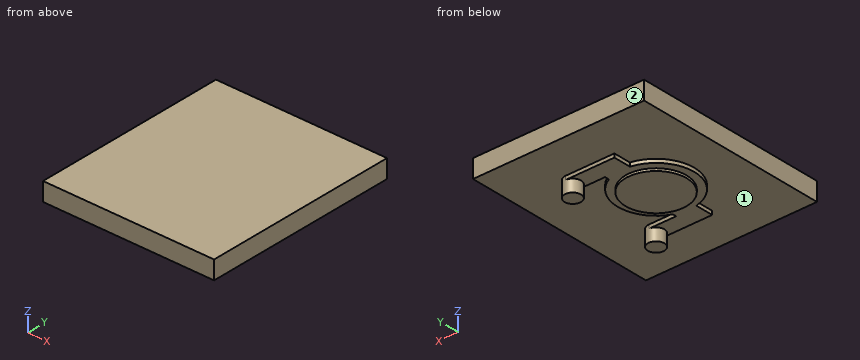
Autodesk Inventor part; units mm, degrees
ref_plane "Work Plane2" through (-8.091, -6.214, -0.6) normal (0, 0, 1) x (1, 0, 0)
ref_plane "Work Plane3" through (-9, -11.7, -1) normal (0, 0, -1) x (0, 1, 0)
ref_plane "YZ Plane" through (0, 0, 0) normal (1, 0, 0) x (0, 1, 0)
ref_plane "Work Plane1" through (0, 0, 0) normal (0, 0, 1) x (1, 0, 0)
sketch "Sketch1" plane through (0, 0, 0) normal (0, 0, 1) x (1, 0, 0)
  line L0 (9, 11.7) -> (-9, 11.7)
  line L1 (-9, 11.7) -> (-9, -11.7)
  line L2 (-9, -11.7) -> (9, -11.7)
  line L3 (9, -11.7) -> (9, 11.7)
  line L4 (5, -9.05) -> (-2.9937, -9.05)
  line L5 (-2.9937, -9.05) -> (-2.9937, -6.1068)
  arc A0 (-2.9937, 6.1788) -> (-2.9937, -6.1068) centre (-1.841, 0.036) ccw
  line L6 (-2.9937, 6.1788) -> (-2.9937, 9.05)
  line L7 (-2.9937, 9.05) -> (5, 9.05)
  arc A1 (5, 6.35) -> (5, 9.05) centre (5, 7.7) ccw
  line L8 (5, 6.35) -> (0.9246, 6.35)
  line L9 (0.9246, 6.35) -> (0.9246, 5.6409)
  arc A2 (0.5216, -5.7502) -> (0.9246, 5.6409) centre (-1.841, 0.036) ccw
  line L10 (0.5216, -5.7502) -> (0.5216, -6.35)
  line L11 (0.5216, -6.35) -> (5, -6.35)
  arc A3 (5, -9.05) -> (5, -6.35) centre (5, -7.7) ccw
  line L12 (-14, -16) -> (14, -16)
  line L13 (14, -16) -> (14, 16)
  line L14 (14, 16) -> (-14, 16)
  line L15 (-14, 16) -> (-14, -16)
  line L16 (-14, -16) -> (14, 16) construction
  line L17 (14, -16) -> (-14, 16) construction
  point P0 (0, 0)
  dimension "d0" = 28
  dimension "d1" = 32
extrude "Extrusion1" add sketch "Sketch1" along normal blind 3 contours L3 L2 L1 L0 | L4 L5 A0 L6 L7 A1 L8 L9 A2 L10 L11 A3 | L15 L14 L13 L12
sketch "Sketch2" plane through (0, 0, 0) normal (0, 0, -1) x (-1, 0, 0)
  circle A0 centre (1.841, 0.036) radius 6.25
  arc A1 (-5, -9.05) -> (-5, -6.35) centre (-5, -7.7) ccw
  line L0 (-0.5216, -6.35) -> (-5, -6.35)
  line L1 (-0.5216, -5.7502) -> (-0.5216, -6.35)
  arc A2 (-0.5216, -5.7502) -> (2.9937, -6.1068) centre (1.841, 0.036) ccw
  line L2 (2.9937, -9.05) -> (2.9937, -6.1068)
  line L3 (-5, -9.05) -> (2.9937, -9.05)
  arc A3 (2.9937, 6.1788) -> (-0.9246, 5.6409) centre (1.841, 0.036) ccw
  line L4 (-0.9246, 6.35) -> (-0.9246, 5.6409)
  line L5 (-5, 6.35) -> (-0.9246, 6.35)
  arc A4 (-5, 6.35) -> (-5, 9.05) centre (-5, 7.7) ccw
  line L6 (2.9937, 9.05) -> (-5, 9.05)
  line L7 (2.9937, 6.1788) -> (2.9937, 9.05)
  circle A5 centre (-5, 7.7) radius 1.35
  circle A6 centre (-5, -7.7) radius 1.35
  point P0 (0, 0)
ref_plane "Work Plane2" through (-8.091, -6.214, -0.6) normal (0, 0, 1) x (1, 0, 0)
extrude "Extrusion2" add sketch "Sketch2" along normal up to surface (0.6 mm away)
sketch "Sketch3" plane through (5, -9.05, -0.6) normal (0, 0, -1) x (-1, 0, 0)
  circle A0 centre (6.841, 9.086) radius 5
  circle A1 centre (0, 16.75) radius 1.35
  circle A2 centre (0, 1.35) radius 1.35
  point P0 (5, 9.05)
extrude "Extrusion3" add sketch "Sketch3" along normal blind 2
sketch "Sketch4" plane through (-1.841, 0.036, -2.6) normal (0, 0, -1) x (-1, 0, 0)
  circle A0 centre (0, 0) radius 5.2
  point P0 (-1.841, -0.036)
ref_plane "Work Plane3" through (-9, -11.7, -1) normal (0, 0, -1) x (0, 1, 0)
extrude "Extrusion4" cut sketch "Sketch4" against normal up to surface (1.6 mm away)
properties part number "00_PDMS_mould_0"
Part model, mm, in its own coordinate system. Face numbers are marked on the shaded views. A direction names the side the tool comes from. Coordinates: 2 decimals unless noted, no trailing zeros. Write each loop counter-clockwise with the first axis right and the second up, starting at its lowest first coordinate (ties: lowest second). Pieces come first, ordered by that corner, then holes. Notation, with made-up numbers: (-17.5, -3.75) - (12.5, -3.75) arc R25 cw to (12.5, 11.25) - close; hole circle Ø2 at (-3, -12.75). An arc over 180 degrees is marked (long way). Put each result on its own line as item: value.
1. Band-saw the part on A-A (y = -7.7). Write the cut outline in (x, z).
Final values:
outline: (-14, 0) - (-2.99, 0) - (-2.99, -0.6) - (3.65, -0.6) - (3.65, -2.6) - (6.35, -2.6) - (6.35, 0) - (14, 0) - (14, 3) - (-14, 3) - close
2. Probe line 1 along Z through (x, y) = (-12.5, 14); line 2 along Z through (x, y) = (-1, -0.5); line 3 along X through (y, z) = (7.5, -1.5). List the from-to ranges inside material, lowest first. Write a range as [from, to].
Final values:
line 1: z = [0, 3]
line 2: z = [-1, 3]
line 3: x = [3.66, 6.34]
3. Band-saw the part on C-C (x = -6.25). Write the cut outline in (y, z).
Final values:
outline: (-16, 0) - (-4.39, 0) - (-4.39, -0.6) - (-2.32, -0.6) - (-2.32, -1) - (2.39, -1) - (2.39, -0.6) - (4.47, -0.6) - (4.47, 0) - (16, 0) - (16, 3) - (-16, 3) - close
4. Band-saw the part on B-B (z = -1.4). Write the cut outline in (x, y), then the cut area to 3 significant figures.
Final values:
outline: circle Ø2.7 at (5, -7.7); circle Ø2.7 at (5, 7.7)
area: 11.5 mm²
5. Flat gauge pins, fed straight in: pin 1 Ø0.5 at (x, z) = (-0.5, -0.5) entering from -Y; pin 2 Ø3 at (x, y) = (0, 2) entering from -Z; pin 3 Ø0.7 at (y, z) = (-7.5, -0.5) entering from -X. Where does each tip first touch, or does it go through?
Final values:
pin 1: stops at y = -9.05
pin 2: stops at z = -1
pin 3: stops at x = -2.99
6. Band-saw the part on D-D (y = -2). Write the cut outline in (x, z).
Final values:
outline: (-14, 0) - (-7.75, 0) - (-7.75, -0.6) - (-6.41, -0.6) - (-6.41, -1) - (2.73, -1) - (2.73, -0.6) - (4.07, -0.6) - (4.07, 0) - (14, 0) - (14, 3) - (-14, 3) - close
7. 3-axis set-ups, long thin cutter, end or side, ignore diameter. For the marked faces 1 and 2: which of +Z, -Z, +X, -X, +Y, -Y reach the whole face in a straight line?
Final values:
face 1: -Z
face 2: +Z, -Z, +X, -X, +Y
